Check sheet for the modelled part. Datum: model origin and axes. Units: mm. Face numbers are marked on the shaded views. A direction names the side the tool comes from. Round coordinates to 2 decimals unless told otherwise and drop trailing zeros. Loops run counter-clockwise (first coordinate to the right, second up) from the corner with the lowest first, then second, coordinate; pieces in that order, holes last. Notation, with made-up numbers: (20.25, -4) - (38.25, -4) arc R20 ccw to (38.25, 14) - close; hole circle Ø7 at (65, 86.5). An arc over 180 degrees is marked (long way). Answer in a Markdown table with one row per item. Add a question column.
(1) Access from +Z, -Z, +X, -X, +Y, -Y to the whole of each face (thin tool, end or side, straight path). Record for the marked faces 4, 5 and 6.
(2) Cross-section at D-D on x = 23. Enter the section's corners in (y, z).
(3) Cross-section at C-C on x = 73.5. Enter the section's corners in (y, z).
(4) Cross-section at B-B on y = 13.75. Enter the section's corners in (x, z).
(5) Gauge pin test, flat ends, axial feed: pin 1 (5 mm diameter, centred on y = 3.5, z = 6.5, fed in from +X); pin 2 (3 mm diameter, centred on y = 6.5, z = 36.5, fed in from +X); pin 3 (11 mm diameter, centred on y = 14.5, z = 5.5, fed in from +X). Record the tip position at first contact, or that the pin passes through.
(6) Mould release check, pull along X, two halves, no side actions. Record for the marked faces 1, 2 and 3: +X half, -X half, draft (parallel to the pull), parting line (faces both ways), or undercut.
(7) Thickness scan on line 1 along X through (y, z) = (6.5, 20); line 2 along Z through (x, y) = (70, 5); line 3 along X through (y, z) = (7.25, 21). Record the ranges inside material, lowest first.
(8) Cross-section at A-A on z = 20. Enter the section's corners in (x, y).
Autodesk Fusion 360 part; units mm, degrees
sketch "Sketch1" plane through (0, 0, 0) normal (0, 1, 0) x (1, 0, 0)
  line L0 (50, 0) -> (50, -40)
  line L1 (0, -40) -> (0, 0)
  line L2 (0, 0) -> (20, 0)
  line L3 (30, 0) -> (30, -10)
  line L4 (30, -10) -> (20, -10)
  line L5 (20, -10) -> (20, 0)
  line L6 (0, 0) -> (20, 0)
  line L7 (30, 0) -> (50, 0)
  line L8 (30, -40) -> (30, -30)
  line L9 (30, -30) -> (20, -30)
  line L10 (20, -30) -> (20, -40)
  line L11 (50, -40) -> (30, -40)
  line L12 (20, -40) -> (0, -40)
  circle A0 centre (70, -20) radius 20
  line L13 (50, 0) -> (70, 0)
  line L14 (50, -40) -> (70, -40)
  circle A1 centre (70, -20) radius 10
  dimension "d1" = 50
  dimension "d2" = 40
  dimension "d3" = 20
  dimension "d4" = 10
  dimension "d5" = 10
  dimension "d6" = 20
  dimension "d7" = 10
  dimension "d8" = 10
  dimension "d9" = 20
extrude "Extrude1" add sketch "Sketch1" along normal blind 20
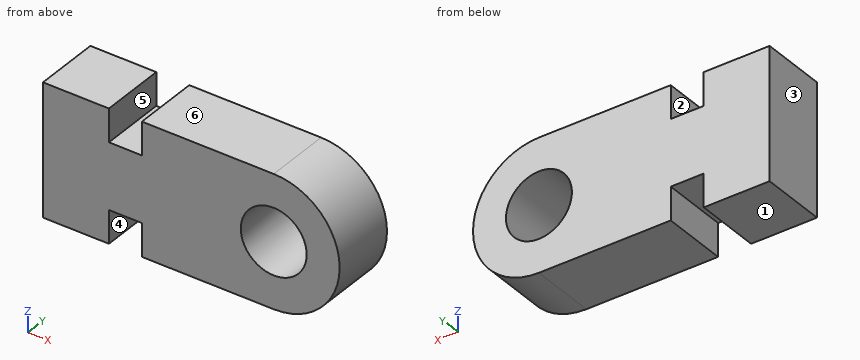
Answers:
| question | item | result |
|---|---|---|
| 1 | face 4 | -Z, +Y, -Y |
| 1 | face 5 | +Z, +Y, -Y |
| 1 | face 6 | +Z, +X, -X, +Y, -Y |
| 2 | outline | (0, 10) - (20, 10) - (20, 30) - (0, 30) - close |
| 3 | outline | (0, 0.31) - (20, 0.31) - (20, 10.63) - (0, 10.63) - close; (0, 29.37) - (20, 29.37) - (20, 39.69) - (0, 39.69) - close |
| 4 | outline | (0, 0) - (20, 0) - (20, 10) - (30, 10) - (30, 0) - (70, 0) arc R20 ccw to (70, 40) - (30, 40) - (30, 30) - (20, 30) - (20, 40) - (0, 40) - close; hole circle Ø20 at (70, 20) |
| 5 | pin 1 | stops at x = 86.7 |
| 5 | pin 2 | stops at x = 83.23 |
| 5 | pin 3 | stops at x = 87.86 |
| 6 | face 1 | draft |
| 6 | face 2 | undercut |
| 6 | face 3 | -X half |
| 7 | line 1 | x = 0 to 60, 80 to 90 |
| 7 | line 2 | z = 0 to 10, 30 to 40 |
| 7 | line 3 | x = 0 to 60.05, 79.95 to 89.97 |
| 8 | outline | (0, 0) - (60, 0) - (60, 20) - (0, 20) - close; (80, 0) - (90, 0) - (90, 20) - (80, 20) - close |
